For this review, take the finished solid that the model builds, in its own axes (mm). Face numbers are marked on the shaded views. A direction names the side the tool comes from. Round coordinates to 2 decimals unless told otherwise and drop trailing zeros. Write each loop counter-clockwise with the first axis right and the second up, starting at its lowest first coordinate (ties: lowest second). Pieces come first, ordered by that corner, then holes. Notation, with made-up numbers: (73.5, 68) -> (99.5, 68) arc R30 ccw to (99.5, 106) -> close; hole circle Ø9 at (82, 61). An arc over 180 degrees is marked (long way). Answer as CSV lines item,"result". Start each with the question number.
Item 1: For pin 1 Ø0.8 at (x, y) = (-16.5, -3) entering from +Z; pin 2 Ø3 at (x, y) = (-9, -0.5) entering from +Z; pin 3 Ø1 at (y, z) = (3.5, -1) entering from -X; pin 4 Ø2 at (x, z) = (-23, -0.5) entering from +Y, all flat-tipped, find the tip position at first contact; note any pin that passes through.
Item 2: Machinability: for the marked faces 5, 6, 7, 8 and 9, which of the approach directions +Z, -Z, +X, -X, +Y, -Y give a long, thin tool a straight path to every point of the face, cutting with its end or side? Answer none if there is none.
Item 3: Take a section at B-B on x = -11.5. Give the boundary of the cut face in (y, z), then the cut area to 3 significant figures.
Item 4: Mouldability with a two-part tool opening along X and no side actions: class the marked faces 1, 2, 3 and 4 as +X half, -X half, draft (parallel to the pull), parting line (faces both ways), or undercut.
Item 5: Wall thickness on probe 1 along Z at (x, y) = (-9.75, 0); probe 2 along Z at (x, y) = (-22.5, 1.5); probe 3 along Y at (x, z) = (-23.5, -2.5): over which ranges is each line inside the solid? List them lowest first. Write a range as from..to.
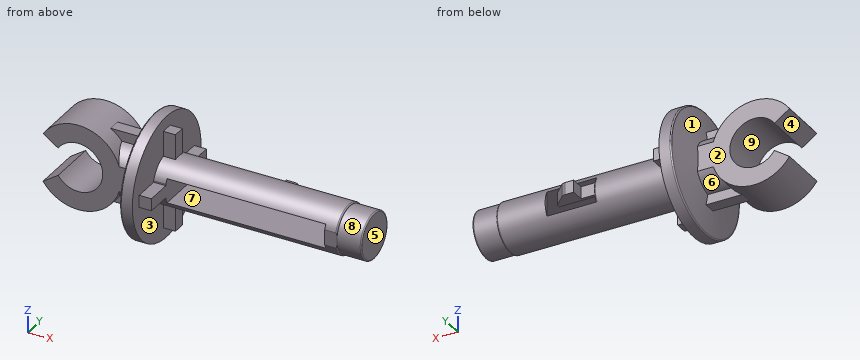
```python
from build123d import *

# Parameters (mm, degrees)
SCHIZZO1_R                    = 2
ESTRUSIONE_ESTRUSIONE1_DEPTH  = 17
SCHIZZO2_OUTSIDE_W            = 9.584
SCHIZZO2_OUTSIDE_H            = 9.584
SCHIZZO2_OUTSIDE_R            = 1.9
TAGLIO_ESTRUSIONE1_DEPTH      = 2
SCHIZZO6_W                    = 15
SCHIZZO6_H                    = 4
TAGLIO_ESTRUSIONE3_DEPTH      = 0.1
TAGLIO_ESTRUSIONE4_DEPTH      = 1.7
TAGLIO_ESTRUSIONE4_DEPTH_BACK = 18.23368794
SCHIZZO5_W                    = 13
SCHIZZO5_H                    = 2
SCHIZZO7_W                    = 4
SCHIZZO7_H                    = 2
TAGLIO_ESTRUSIONE5_DEPTH      = 18.555910686
ESTRUSIONE_ESTRUSIONE2_DEPTH  = 0.5
TAGLIO_ESTRUSIONE6_DEPTH      = 0.07
ESTRUSIONE_ESTRUSIONE4_DEPTH  = 0.5
ESTRUSIONE_ESTRUSIONE5_DEPTH  = 0.5
SCHIZZO20_R                   = 5
ESTRUSIONE_ESTRUSIONE6_DEPTH  = 1
SCHIZZO23_R                   = 2.25
ESTRUSIONE_ESTRUSIONE7_DEPTH  = 3
ESTRUSIONE_ESTRUSIONE10_DEPTH = 2
ESTRUSIONE_ESTRUSIONE8_DEPTH  = 0.5
SCHIZZO35_W                   = 3
SCHIZZO35_H                   = 2.061552812
TAGLIO_ESTRUSIONE7_DEPTH      = 1
RACCORDO22_R                  = 0.5
RACCORDO23_R                  = 0.1
RACCORDO24_R                  = 0.1
RACCORDO25_R                  = 0.1
RACCORDO28_R                  = 0.1


# Some blends are built 0.0001 mm under size
with BuildPart() as part:
    # Schizzo1 → Estrusione-Estrusione1 (new body)
    with BuildSketch(Plane(origin=(0, 0, 0), x_dir=(0, 0, -1), z_dir=(1, 0, 0))):
        Circle(SCHIZZO1_R)
    extrude(amount=-ESTRUSIONE_ESTRUSIONE1_DEPTH)

    # Schizzo2 outside → Taglio-Estrusione1 (cut)
    with BuildSketch(Plane(origin=(0, 0, 0), x_dir=(0, 0, -1), z_dir=(1, 0, 0))):
        Rectangle(SCHIZZO2_OUTSIDE_W, SCHIZZO2_OUTSIDE_H)
        Circle(SCHIZZO2_OUTSIDE_R, mode=Mode.SUBTRACT)
    extrude(amount=-TAGLIO_ESTRUSIONE1_DEPTH, mode=Mode.SUBTRACT)

    # Schizzo6 → Taglio-Estrusione3 (cut)
    with BuildSketch(Plane(origin=(0, -2, 0), x_dir=(-1, 0, 0), z_dir=(0, -1, 0))):
        with Locations((9.5, 0)):
            Rectangle(SCHIZZO6_W, SCHIZZO6_H)
    extrude(amount=-TAGLIO_ESTRUSIONE3_DEPTH, mode=Mode.SUBTRACT)

    # Schizzo5 → Taglio-Estrusione4 (cut, two sides: drawn at the far end of the back side and taken through both)
    with BuildSketch(Plane(origin=(0, 0, 0), x_dir=(1, 0, 0), z_dir=(0, 1, 0)).offset(-TAGLIO_ESTRUSIONE4_DEPTH_BACK)):
        with Locations((-9.5, 0)):
            Rectangle(SCHIZZO5_W, SCHIZZO5_H)
    extrude(amount=TAGLIO_ESTRUSIONE4_DEPTH + TAGLIO_ESTRUSIONE4_DEPTH_BACK, mode=Mode.SUBTRACT)

    # Schizzo7 → Taglio-Estrusione5 (cut, through all)
    with BuildSketch(Plane(origin=(0, 2, 0), x_dir=(1, 0, 0), z_dir=(0, 1, 0))):
        with Locations((-8, 0)):
            Rectangle(SCHIZZO7_W, SCHIZZO7_H)
    extrude(amount=-TAGLIO_ESTRUSIONE5_DEPTH, mode=Mode.SUBTRACT)

    # Schizzo12 → Estrusione-Estrusione2 (add, symmetric)
    with BuildSketch(Plane.XY):
        Polygon((-10, 2), (-8.9, 2), (-8.9, 3), (-8, 3), (-7, 2), (-7, 1.7), (-10, 1.7), align=None)
    extrude(amount=ESTRUSIONE_ESTRUSIONE2_DEPTH, both=True)

    # Schizzo16 → Taglio-Estrusione6 (cut)
    with BuildSketch(Plane(origin=(0, 2, 0), x_dir=(1, 0, 0), z_dir=(0, 1, 0))):
        Polygon((-8.9, 0.5), (-10, 0.5), (-10, 0), (-10, -0.5), (-8.9, -0.5), align=None)
    extrude(amount=-TAGLIO_ESTRUSIONE6_DEPTH, mode=Mode.SUBTRACT)

    # Schizzo17 → Estrusione-Estrusione4 (add, symmetric)
    with BuildSketch(Plane.XY):
        Polygon((-17, 4), (-16, 4), (-16, 0.047058824), (-17, 0.05), align=None)
    estrusione_estrusione4 = extrude(amount=ESTRUSIONE_ESTRUSIONE4_DEPTH, both=True)

    # Specchia2: Estrusione-Estrusione4 across plane
    add(estrusione_estrusione4.mirror(Plane.ZX))

    # Schizzo19 → Estrusione-Estrusione5 (add, symmetric)
    with BuildSketch(Plane(origin=(0, 0, 0), x_dir=(1, 0, 0), z_dir=(0, 1, 0))):
        Polygon((-17, 2), (-17, 0), (-16, 0), (-16, 2), (-16, 4), (-17, 4), align=None)
    estrusione_estrusione5 = extrude(amount=ESTRUSIONE_ESTRUSIONE5_DEPTH, both=True)

    # Specchia5: Estrusione-Estrusione5 across plane
    add(estrusione_estrusione5.mirror(Plane.XY))

    # Schizzo20 → Estrusione-Estrusione6 (add)
    with BuildSketch(Plane.ZY.offset(17)):
        Circle(SCHIZZO20_R)
    extrude(amount=ESTRUSIONE_ESTRUSIONE6_DEPTH)

    # Schizzo23 → Estrusione-Estrusione7 (add)
    with BuildSketch(Plane.ZY.offset(18)):
        Circle(SCHIZZO23_R)
    extrude(amount=ESTRUSIONE_ESTRUSIONE7_DEPTH)

    # Schizzo22 → Estrusione-Estrusione10 (add, symmetric)
    with BuildSketch(Plane(origin=(0, 0, 0), x_dir=(1, 0, 0), z_dir=(0, 1, 0))):
        with BuildLine():
            Line((-24.762298216, -1.129872594), (-26, -1.977277039))
            ThreePointArc((-26, -1.977277039), (-19.612029171, 0), (-26, 1.977277039))
            Line((-26, 1.977277039), (-24.762298216, 1.129872594))
            ThreePointArc((-24.762298216, 1.129872594), (-21.112029171, 0), (-24.762298216, -1.129872594))
        make_face()
    extrude(amount=ESTRUSIONE_ESTRUSIONE10_DEPTH, both=True)

    # Schizzo34 → Estrusione-Estrusione8 (add, symmetric)
    with BuildSketch(Plane(origin=(0, 0, 0), x_dir=(1, 0, 0), z_dir=(0, 1, 0))):
        Polygon((-18, 3), (-21.309253533, 3), (-18, 0), align=None)
    estrusione_estrusione8 = extrude(amount=ESTRUSIONE_ESTRUSIONE8_DEPTH, both=True)

    # Specchia6: Estrusione-Estrusione8 across plane
    add(estrusione_estrusione8.mirror(Plane.XY))

    # Schizzo35 → Taglio-Estrusione7 (cut)
    with BuildSketch(Plane(origin=(0, 2, 0), x_dir=(1, 0, 0), z_dir=(0, 1, 0))):
        with Locations((-19.5, 0)):
            Rectangle(SCHIZZO35_W, SCHIZZO35_H)
    taglio_estrusione7 = extrude(amount=TAGLIO_ESTRUSIONE7_DEPTH, mode=Mode.SUBTRACT)

    # Specchia7: Taglio-Estrusione7 across plane
    add(taglio_estrusione7.mirror(Plane.ZX), mode=Mode.SUBTRACT)

    # Raccordo22
    raccordo22_edges = [part.edges().sort_by_distance(p)[0] for p in [
        (-8, 3, 0),
    ]]
    fillet(raccordo22_edges, radius=RACCORDO22_R)

    # Raccordo23
    raccordo23_edges = [part.edges().sort_by_distance(p)[0] for p in [
        (-2, 2, 0),
    ]]
    fillet(raccordo23_edges, radius=RACCORDO23_R - 0.0001)  # a hair under: the kernel refuses the full size

    # Raccordo24
    raccordo24_edges = [part.edges().sort_by_distance(p)[0] for p in [
        (0, 0, 1.9),
    ]]
    fillet(raccordo24_edges, radius=RACCORDO24_R)

    # Raccordo25
    raccordo25_edges = [part.edges().sort_by_distance(p)[0] for p in [
        (-18, 0, -5),
    ]]
    fillet(raccordo25_edges, radius=RACCORDO25_R)

    # Raccordo28
    # the kernel refuses this fillet: 0.1 mm, written as the material it takes off along each edge
    with BuildSketch(Plane(origin=(-10, 0, 0), x_dir=(0, 0.7969175395012055, 0.6040881022130338), z_dir=(0, -0.6040881022130338, 0.7969175395012055))) as raccordo28_piece_1_section:
        with BuildLine():
            CenterArc((2 - RACCORDO28_R, RACCORDO28_R), RACCORDO28_R, 270, 90)
            Line((2 - RACCORDO28_R, 0), (2, 0))
            Line((2, 0), (2, RACCORDO28_R))
        make_face()
    raccordo28_piece_1 = revolve(axis=Axis((-10, 0, 0), (-1, 0, 0)), revolution_arc=74.326501832, mode=Mode.PRIVATE)
    raccordo28_piece_1 = split(raccordo28_piece_1, bisect_by=Plane(origin=(-10.022414525, 1.819827674, 1), z_dir=(0, 0, -1)), keep=Keep.TOP, mode=Mode.PRIVATE)
    raccordo28_piece_1 = split(raccordo28_piece_1, bisect_by=Plane(origin=(-10.022414525, 1.819827674, 0.5), z_dir=(0, 0, 1)), keep=Keep.TOP, mode=Mode.PRIVATE)
    raccordo28_piece_1 = split(raccordo28_piece_1, bisect_by=Plane(origin=(-10.022414525, 1.93, 0.756995565), z_dir=(0, -1, 0)), keep=Keep.TOP, mode=Mode.PRIVATE)
    add(raccordo28_piece_1, mode=Mode.SUBTRACT)
    with BuildSketch(Plane(origin=(-10, 0, 0), x_dir=(0, 0.7969175395012055, 0.6040881022130338), z_dir=(0, -0.6040881022130338, 0.7969175395012055))) as raccordo28_piece_2_section:
        with BuildLine():
            CenterArc((2 - RACCORDO28_R, RACCORDO28_R), RACCORDO28_R, 270, 90)
            Line((2 - RACCORDO28_R, 0), (2, 0))
            Line((2, 0), (2, RACCORDO28_R))
        make_face()
    raccordo28_piece_2 = revolve(axis=Axis((-10, 0, 0), (-1, 0, 0)), revolution_arc=74.326501832, mode=Mode.PRIVATE)
    raccordo28_piece_2 = split(raccordo28_piece_2, bisect_by=Plane(origin=(-10.044225117, 1.932988234, 0.5), z_dir=(0, 0, 1)), keep=Keep.TOP, mode=Mode.PRIVATE)
    raccordo28_piece_2 = split(raccordo28_piece_2, bisect_by=Plane(origin=(-10.044225117, 1.93, 0.511192028), z_dir=(0, 1, 0)), keep=Keep.TOP, mode=Mode.PRIVATE)
    add(raccordo28_piece_2, mode=Mode.SUBTRACT)
    with BuildSketch(Plane(origin=(-10, 0, 0), x_dir=(0, 0.7969175395012055, 0.6040881022130338), z_dir=(0, -0.6040881022130338, 0.7969175395012055))) as raccordo28_piece_3_section:
        with BuildLine():
            CenterArc((2 - RACCORDO28_R, RACCORDO28_R), RACCORDO28_R, 270, 90)
            Line((2 - RACCORDO28_R, 0), (2, 0))
            Line((2, 0), (2, RACCORDO28_R))
        make_face()
    raccordo28_piece_3 = revolve(axis=Axis((-10, 0, 0), (-1, 0, 0)), revolution_arc=74.326501832, mode=Mode.PRIVATE)
    raccordo28_piece_3 = split(raccordo28_piece_3, bisect_by=Plane(origin=(-10.022414524, 1.819827674, -1), z_dir=(0, 0, 1)), keep=Keep.TOP, mode=Mode.PRIVATE)
    raccordo28_piece_3 = split(raccordo28_piece_3, bisect_by=Plane(origin=(-10.022414524, 1.93, -0.756995565), z_dir=(0, -1, 0)), keep=Keep.TOP, mode=Mode.PRIVATE)
    raccordo28_piece_3 = split(raccordo28_piece_3, bisect_by=Plane(origin=(-10.022414524, 1.819827674, -0.5), z_dir=(0, 0, -1)), keep=Keep.TOP, mode=Mode.PRIVATE)
    add(raccordo28_piece_3, mode=Mode.SUBTRACT)
    with BuildSketch(Plane(origin=(-10, 0, 0), x_dir=(0, 0.7969175395012055, 0.6040881022130338), z_dir=(0, -0.6040881022130338, 0.7969175395012055))) as raccordo28_piece_4_section:
        with BuildLine():
            CenterArc((2 - RACCORDO28_R, RACCORDO28_R), RACCORDO28_R, 270, 90)
            Line((2 - RACCORDO28_R, 0), (2, 0))
            Line((2, 0), (2, RACCORDO28_R))
        make_face()
    raccordo28_piece_4 = revolve(axis=Axis((-10, 0, 0), (-1, 0, 0)), revolution_arc=74.326501832, mode=Mode.PRIVATE)
    raccordo28_piece_4 = split(raccordo28_piece_4, bisect_by=Plane(origin=(-10.040080162, 1.981654904, 0.5), z_dir=(0, 0, -1)), keep=Keep.TOP, mode=Mode.PRIVATE)
    raccordo28_piece_4 = split(raccordo28_piece_4, bisect_by=Plane(origin=(-10.040080162, 1.93, 0), z_dir=(0, 1, 0)), keep=Keep.TOP, mode=Mode.PRIVATE)
    raccordo28_piece_4 = split(raccordo28_piece_4, bisect_by=Plane(origin=(-10.040080162, 1.981654904, -0.5), z_dir=(0, 0, 1)), keep=Keep.TOP, mode=Mode.PRIVATE)
    add(raccordo28_piece_4, mode=Mode.SUBTRACT)
    with BuildSketch(Plane(origin=(-10, 0, 0), x_dir=(0, 0.7969175395012055, 0.6040881022130338), z_dir=(0, -0.6040881022130338, 0.7969175395012055))) as raccordo28_piece_5_section:
        with BuildLine():
            CenterArc((2 - RACCORDO28_R, RACCORDO28_R), RACCORDO28_R, 270, 90)
            Line((2 - RACCORDO28_R, 0), (2, 0))
            Line((2, 0), (2, RACCORDO28_R))
        make_face()
    raccordo28_piece_5 = revolve(axis=Axis((-10, 0, 0), (-1, 0, 0)), revolution_arc=74.326501832, mode=Mode.PRIVATE)
    raccordo28_piece_5 = split(raccordo28_piece_5, bisect_by=Plane(origin=(-10.044225117, 1.93, -0.511192028), z_dir=(0, 1, 0)), keep=Keep.TOP, mode=Mode.PRIVATE)
    raccordo28_piece_5 = split(raccordo28_piece_5, bisect_by=Plane(origin=(-10.044225117, 1.932988234, -0.5), z_dir=(0, 0, -1)), keep=Keep.TOP, mode=Mode.PRIVATE)
    add(raccordo28_piece_5, mode=Mode.SUBTRACT)

    # Estrusione-Estrusione9 cone 1 section (through the dimple's axis) → Estrusione-Estrusione9 (revolve)
    with BuildSketch(Plane(origin=(-18, 0, 0), x_dir=(0, 0, -1), z_dir=(0, 1, 0))):
        Polygon((0, 0), (4.9, 0), (0, 0.864002205), align=None)
    revolve(axis=Axis((-18, 0, 0), (-1, 0, 0)))


solid = part.part
```
Output values:
1,pin 1,"stops at z = 0.5"
1,pin 2,"stops at z = 2"
1,pin 3,"stops at x = -18.31"
1,pin 4,"passes through"
2,face 5,"+Z, -Z, +X, +Y, -Y"
2,face 6,"-Z, +Y"
2,face 7,"-Y"
2,face 8,"+X"
2,face 9,"+Y, -Y"
3,outline,"(-1.73, -1) arc R2 ccw (long way) to (-1.73, 1) -> (1.7, 1) -> (1.7, -1) -> close"
3,area,"5.34 mm^2"
4,face 1,"undercut"
4,face 2,"draft"
4,face 3,"+X half"
4,face 4,"-X half"
5,probe 1,"z = -2..-1, 1..2"
5,probe 2,"z = -3.45..-1.9, 1.9..3.45"
5,probe 3,"y = -2..2"
